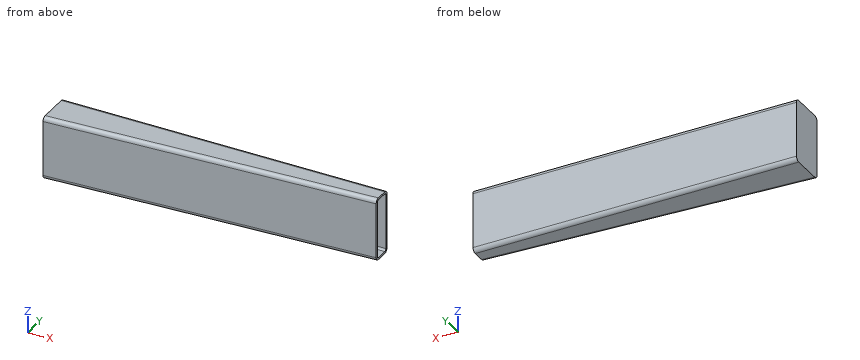
from build123d import *

# Parameters (mm, degrees)
SKETCH1_W           = 410
SKETCH1_H           = 80.00000002
BOSS_EXTRUDE1_DEPTH = 65
CUT_EXTRUDE1_DEPTH  = 96.52
FILLET1_R           = 5.08
FILLET2_R           = 5.08
FILLET3_R           = 5.08
FILLET4_R           = 5.08
SHELL2_T            = -2.54


with BuildPart() as part:
    # Sketch1 → Boss-Extrude1 (new body)
    with BuildSketch(Plane(origin=(0, 0, 0), x_dir=(1, 0, 0), z_dir=(0, 1, 0))):
        with Locations((201.324966403, -38.031873554)):
            Rectangle(SKETCH1_W, SKETCH1_H)
    extrude(amount=BOSS_EXTRUDE1_DEPTH)

    # Sketch3 → Cut-Extrude1 (cut)
    with BuildSketch(Plane.XY.offset(78.031873564)):
        Polygon((-3.675033597, 17.620000018), (406.324966403, 40), (452.471299635, -78.145402135), (-12.284026323, -65.583685792), (-43.531224316, 90.933184559), align=None)
    extrude(amount=-CUT_EXTRUDE1_DEPTH, mode=Mode.SUBTRACT)

    # Fillet1
    fillet1_edges = [part.edges().sort_by_distance(p)[0] for p in [
        (201.324966403, 65, 78.031873564),
    ]]
    fillet(fillet1_edges, radius=FILLET1_R)

    # Fillet2
    fillet2_edges = [part.edges().sort_by_distance(p)[0] for p in [
        (201.324966403, 28.810000009, 78.031873564),
    ]]
    fillet(fillet2_edges, radius=FILLET2_R)

    # Fillet3
    fillet3_edges = [part.edges().sort_by_distance(p)[0] for p in [
        (201.324966403, 65, -1.968126456),
    ]]
    fillet(fillet3_edges, radius=FILLET3_R)

    # Fillet4
    fillet4_edges = [part.edges().sort_by_distance(p)[0] for p in [
        (201.324966403, 28.810000009, -1.968126456),
    ]]
    fillet(fillet4_edges, radius=FILLET4_R)

    # Shell2
    shell2_openings = [part.faces().sort_by_distance(p)[0] for p in [
        (406.324966403, 52.501499056, 38.031873554),
    ]]
    offset(amount=SHELL2_T, openings=shell2_openings, kind=Kind.INTERSECTION)


solid = part.part
Input: part model. Units: mm. Frame: model coordinates. Give positions to 0.01 mm unless a question says otherwise; leave off trailing zeros. Write each loop counter-clockwise with the first axis right and the second up, starting at its lowest first coordinate (ties: lowest second). Pieces come first, ordered by that corner, then holes. Notation, with made-up numbers: M 36.5,49 L 70.5,49 A20 cw 70.5,60 Z; hole C 27,-0.5 d11. An arc over 180 degrees is marked long. Write item = value, one per line. Start each with the question number.
1) Material intervals for line 1 along Z through (x, y) = (250, 58.5); line 2 along X through (y, z) = (56.5, 40.5); line 3 along Y through (x, z) = (251, 63), sorted ascending. Write a range as [from, to].
2) First-contact query: pin 1 Ø21 at (x, z) = (216.5, 50) entering from -Y; pin 2 Ø6 at (x, z) = (286, 8.5) entering from -Y; pin 3 Ø6 at (x, y) = (192.5, 29) entering from +Z. Flat tips, straight axial feed; report the tip coordinate or a pass-through.
3) Cut plane A-A on z = 37. Return the cut outline in (x, y), then the cut area to 3 significant figures.
4) Cut plane B-B on y = 54.5. Return the cut outline in (x, z).
Solved:
q1.line_1 = [-1.97, 0.57], [75.49, 78.03]
q1.line_2 = [-3.68, -1.14]
q1.line_3 = [31.52, 34.07], [62.46, 65]
q2.pin_1 = 29.07
q2.pin_2 = 33.27
q2.pin_3 = 77.83
q3.outline = M -3.68,17.62 L 406.32,40 L 406.32,42.54 L -1.14,20.3 L -1.14,62.46 L 406.32,62.46 L 406.32,65 L -3.68,65 Z
q3.area = 2,190 mm2
q4.outline = M -3.68,-1.97 L 406.32,-1.97 L 406.32,0.57 L -1.14,0.57 L -1.14,75.49 L 406.32,75.49 L 406.32,78.03 L -3.68,78.03 Z
